For this review, take the finished solid that the model builds, in its own axes (mm). A direction names the side the tool comes from. Give positions to 0.01 mm unless a question says otherwise; leave off trailing zeros. Loops run counter-clockwise (first coordinate to the right, second up) from the corner with the lowest first, then second, coordinate; pieces in that order, holes last. Notation, with made-up numbers: (-1, 15) - (54, 15) arc R22 cw to (54, 27) - close; hole circle Ø11 at (-38, 72). An arc over 180 degrees is marked (long way). Answer in a Markdown table with one row per item.
Autodesk Inventor part; units mm, degrees
ref_plane "YZ Plane" through (0, 0, 0) normal (1, 0, 0) x (0, 1, 0)
ref_plane "XZ Plane" through (0, 0, 0) normal (0, 1, 0) x (-1, 0, 0)
ref_plane "XY Plane" through (0, 0, 0) normal (0, 0, 1) x (1, 0, 0)
sketch "Sketch1" plane through (0, 0, 0) normal (0, 0, 1) x (1, 0, 0)
  line L0 (91, -34) -> (91, 34)
  line L1 (91, 34) -> (41, 34)
  line L2 (41, 34) -> (41, 89)
  line L3 (41, 89) -> (-91, 89)
  line L4 (-91, 89) -> (-91, -89)
  line L5 (-91, -89) -> (41, -89)
  line L6 (41, -89) -> (41, -34)
  line L7 (41, -34) -> (91, -34)
  line L8 (70, 27) -> (62, 27)
  line L9 (91, 34) -> (-87, 34)
  line L10 (-87, 34) -> (-87, 27)
  line L11 (-87, 27) -> (91, 27)
  line L12 (91, 27) -> (91, 34)
  circle A0 centre (-83, 21.5) radius 1.2295
  circle A1 centre (-83, -64.5) radius 1.2295
  circle A2 centre (-83, -21.5) radius 1.2295
  circle A3 centre (-83, 64.5) radius 1.2295
  line L13 (-85, -72) -> (-76, -72)
  line L14 (-76, -72) -> (-76, -57)
  line L15 (-76, -57) -> (-85, -57)
  arc A4 (-87, -55) -> (-85, -57) centre (-85, -55) ccw
  line L16 (-87, -55) -> (-87, -31)
  arc A5 (-85, -29) -> (-87, -31) centre (-85, -31) ccw
  line L17 (-85, -29) -> (-76, -29)
  line L18 (-76, -29) -> (-76, -14)
  line L19 (-76, -14) -> (-85, -14)
  arc A6 (-87, -12) -> (-85, -14) centre (-85, -12) ccw
  line L20 (-87, -12) -> (-87, 12)
  arc A7 (-85, 14) -> (-87, 12) centre (-85, 12) ccw
  line L21 (-85, 14) -> (-76, 14)
  line L22 (-76, 14) -> (-76, 29)
  line L23 (-76, 29) -> (-85, 29)
  arc A8 (-87, 31) -> (-85, 29) centre (-85, 31) ccw
  line L24 (-87, 31) -> (-87, 55)
  arc A9 (-85, 57) -> (-87, 55) centre (-85, 55) ccw
  line L25 (-85, 57) -> (-76, 57)
  line L26 (-76, 57) -> (-76, 72)
  line L27 (-76, 72) -> (-85, 72)
  arc A10 (-87, 74) -> (-85, 72) centre (-85, 74) ccw
  line L28 (-87, 74) -> (-87, 89)
  line L29 (-91, 89) -> (-87, 89)
  line L30 (-91, -89) -> (-91, 89)
  line L31 (-91, -89) -> (-87, -89)
  line L32 (-87, -89) -> (-87, -74)
  arc A11 (-85, -72) -> (-87, -74) centre (-85, -74) ccw
  line L33 (-91, 89.5) -> (-86.5, 89.5)
  line L34 (-86.5, 89.5) -> (-86.5, 74)
  arc A12 (-86.5, 74) -> (-85, 72.5) centre (-85, 74) ccw
  line L35 (-85, 72.5) -> (-75.5, 72.5)
  line L36 (-75.5, 72.5) -> (-75.5, 56.5)
  line L37 (-75.5, 56.5) -> (-85, 56.5)
  arc A13 (-85, 56.5) -> (-86.5, 55) centre (-85, 55) ccw
  line L38 (-86.5, 55) -> (-86.5, 31)
  arc A14 (-86.5, 31) -> (-85, 29.5) centre (-85, 31) ccw
  line L39 (-85, 29.5) -> (-75.5, 29.5)
  line L40 (-75.5, 29.5) -> (-75.5, 13.5)
  line L41 (-75.5, 13.5) -> (-85, 13.5)
  arc A15 (-85, 13.5) -> (-86.5, 12) centre (-85, 12) ccw
  line L42 (-86.5, 12) -> (-86.5, -12)
  arc A16 (-86.5, -12) -> (-85, -13.5) centre (-85, -12) ccw
  line L43 (-85, -13.5) -> (-75.5, -13.5)
  line L44 (-75.5, -13.5) -> (-75.5, -29.5)
  line L45 (-75.5, -29.5) -> (-85, -29.5)
  arc A17 (-85, -29.5) -> (-86.5, -31) centre (-85, -31) ccw
  line L46 (-86.5, -31) -> (-86.5, -55)
  arc A18 (-86.5, -55) -> (-85, -56.5) centre (-85, -55) ccw
  line L47 (-85, -56.5) -> (-75.5, -56.5)
  line L48 (-75.5, -56.5) -> (-75.5, -72.5)
  line L49 (-75.5, -72.5) -> (-85, -72.5)
  arc A19 (-85, -72.5) -> (-86.5, -74) centre (-85, -74) ccw
  line L50 (-86.5, -74) -> (-86.5, -89.5)
  line L51 (-86.5, -89.5) -> (-91, -89.5)
  line L52 (-86.5, 31) -> (-75.5, 31)
  line L53 (-75.5, 31) -> (-75.5, 29.5)
  line L54 (-75.5, 31) -> (-75.5, 34)
  point P0 (0, 0)
  point P1 (-75.5, 27)
  point P2 (-86.5, 34)
  dimension "d6" = 0.5
extrude "Extrusion1" add sketch "Sketch1" along normal blind 30 contours L11 L8 L40 L53 L54 L9 L1 L0
sketch "Sketch3" plane through (-86.5, 34, 0) normal (0, 1, 0) x (1, 0, 0)
  line L0 (-0.5, -4.5) -> (-0.5, 0)
  line L1 (-0.5, 0) -> (-4.5, 0)
  line L2 (-4.5, 0) -> (-4.5, 3.5)
  line L3 (-4.5, 3.5) -> (-18.5, 3.5)
  line L4 (-18.5, 3.5) -> (-4.5, -5.5)
  line L5 (-4.5, -5.5) -> (-4.5, -4.5)
  line L6 (-4.5, -4.5) -> (-0.5, -4.5)
  line L7 (-0.5, -4.5) -> (50.0525, -33.6865)
  line L8 (177.5, 0) -> (11, 0)
  line L9 (177.5, -30) -> (11, -30)
  line L10 (177.5, 0) -> (177.5, -30)
  line L11 (11, 0) -> (11, -30)
  point P0 (86.5, 0)
  point P1 (43.6673, -30)
  point P2 (11, -11.1395)
  dimension "d7" = 30
extrude "Extrusion4" cut sketch "Sketch3" against normal blind 30 contours L7 L9 L11
sketch "Sketch5" plane through (-75.5, 27, 0) normal (0, -1, 0) x (1, 0, 0)
  line L0 (56.5, 7.0341) -> (57.5, 7.0341)
  line L1 (34.5, 7.0341) -> (56.5, 7.0341)
  line L2 (33.5, 7.0341) -> (33.5, 6.6226)
  line L3 (33.5, 6.6226) -> (9.5, 6.6226)
  line L4 (9.5, 6.6226) -> (9.5, 7.0341)
  line L5 (9.5, 7.0341) -> (33.5, 7.0341)
  line L6 (64.5, 7.0341) -> (64.5, 6.6226)
  line L7 (64.5, 6.6226) -> (57.5, 6.6226)
  line L8 (57.5, 6.6226) -> (57.5, 7.0341)
  line L9 (57.5, 7.0341) -> (64.5, 7.0341)
  line L10 (9.5, 2) -> (9.5, 2.6226)
  line L11 (9.5, 2.6226) -> (64.5, 2.6226)
  line L12 (64.5, 2.6226) -> (64.5, 2)
  line L13 (64.5, 2) -> (9.5, 2)
  line L14 (9.5, 7.0341) -> (64.5, 7.0341)
  line L15 (64.5, 7.0341) -> (64.5, 2)
  line L16 (64.5, 2) -> (9.5, 2)
  line L17 (9.5, 2) -> (9.5, 7.0341)
  line L18 (9.2, 7.3341) -> (64.8, 7.3341)
  line L19 (64.8, 7.3341) -> (64.8, 1.9)
  line L20 (64.8, 1.9) -> (9.2, 1.9)
  line L21 (9.2, 1.9) -> (9.2, 7.3341)
  point P0 (75.5, 0)
  dimension "d19" = 0.3
  dimension "d20" = 0.3
  dimension "d21" = 0.1
  dimension "d22" = 0.3
extrude "Extrusion6" cut sketch "Sketch5" against normal blind 0.7 contours L0 L8 L7 L15 L11 L17 L3 L2 L14 L1 | L9 L6 L7 L8 | L2 L3 L4 L5 | L12 L13 L10 L11 | L18 L19 L20 L21
sketch "Sketch6" plane through (-75.5, 27, 0) normal (0, -1, 0) x (1, 0, 0)
  line L0 (33.5, 7.0341) -> (34.5, 7.0341)
  line L1 (34.5, 7.0341) -> (56.5, 7.0341)
  line L2 (56.5, 7.0341) -> (57.5, 7.0341)
  line L3 (64.8, 1.9) -> (9.2, 1.9)
  line L4 (64.8, 7.3341) -> (64.8, 1.9)
  line L5 (9.2, 7.3341) -> (64.8, 7.3341)
  line L6 (9.2, 1.9) -> (9.2, 7.3341)
  line L7 (33.5, 7.3341) -> (57.5, 7.3341)
  line L8 (57.5, 7.3341) -> (57.5, 1.9)
  line L9 (57.5, 1.9) -> (33.5, 1.9)
  line L10 (33.5, 1.9) -> (33.5, 7.3341)
  point P0 (75.5, 0)
extrude "Extrusion7" cut sketch "Sketch6" against normal up to next contours L10 L5 L8 L2 L1 L0 | L0 L1 L2 L8 L3 L10
sketch "Sketch7" plane through (0, 0, 30) normal (0, 0, 1) x (1, 0, 0)
  line L0 (10.25, -34) -> (10.25, 34)
  line L1 (10.25, 34) -> (-5.75, 34)
  line L2 (-5.75, -34) -> (-5.75, 34)
  line L3 (10.25, -34) -> (-5.75, -34)
  line L4 (-42.8327, 27) -> (91, 27)
  line L5 (10.25, 34) -> (-5.75, 34)
  line L6 (-5.75, 34) -> (-5.75, 27)
  line L7 (-5.75, 27) -> (10.25, 27)
  line L8 (10.25, 27) -> (10.25, 34)
  line L9 (10.65, 34) -> (-6.15, 34)
  line L10 (-6.15, 34) -> (-6.15, 27)
  line L11 (-6.15, 27) -> (10.65, 27)
  line L12 (10.65, 27) -> (10.65, 34)
  point P0 (0, 0)
  dimension "d27" = 0.4
  dimension "d28" = 0.4
extrude "Extrusion8" cut sketch "Sketch7" against normal blind 15.5 contours L4 L2 L1 L0 | L0 L9 L12 L4 | L4 L10 L9 L2
properties part number "right_hold"
1. We need section B-B, the plane y = 32.75. Give the boundary of the cut face in (x, z).
Values:
| item | result |
|---|---|
| outline | (-75.5, 0) - (91, 0) - (91, 30) - (10.65, 30) - (10.65, 14.5) - (-6.15, 14.5) - (-6.15, 30) - (-42.83, 30) - (-75.5, 11.14) - close; hole (-42, 1.9) - (-18, 1.9) - (-18, 7.33) - (-42, 7.33) - close |
2. For faces 5 (the face through (-18, 31, 5)), 6 (the face through (-54, 27.7, 5)), 7 (the face through (50, 31, 30)), 8 (the face through (10.65, 30, 22)), list the 3-axis set-ups (+Z, -Z, +X, -X, +Y, -Y) from which the entire face can be reached by the end or side of a thin tool; tool diameter is ignored.
Values:
| item | result |
|---|---|
| face 5 | +Y, -Y |
| face 6 | -Y |
| face 7 | +Z, +X, -X, +Y, -Y |
| face 8 | +Z, +Y, -Y |
3. Clearance check with a flat-ended pin moving along its axis: pin 1 (1.6 mm diameter, centred on x = -13.5, z = 5.5, fed in from -Y). State where the tip first meets the part, or that it passes through.
Values:
| item | result |
|---|---|
| pin 1 | stops at y = 27.7 |
4. We need section C-C, the plane z = 17. Give the boundary of the cut face in (x, y).
Values:
| item | result |
|---|---|
| outline | (-65.35, 27) - (-6.15, 27) - (-6.15, 34) - (-65.35, 34) - close; (10.65, 27) - (91, 27) - (91, 34) - (10.65, 34) - close |
5. Mouldability with a two-part tool opening along Z and no side actions: class faces 1 (the face through (-14, 27.7, 5)), 2 (the face through (-6.15, 31, 22)), 3 (the face through (-59.395, 30.549, 20.438)), 4 (the face through (-33, 30, 7.334)) as released by +Z, released by -Z, zero draft, split by the parting line, or undercut.
Values:
| item | result |
|---|---|
| face 1 | undercut |
| face 2 | zero draft |
| face 3 | released by +Z |
| face 4 | undercut |
6. We need section A-A, the plane x = -31.5. Give the boundary of the cut face in (y, z).
Values:
| item | result |
|---|---|
| outline | (27, 0) - (34, 0) - (34, 1.9) - (27, 1.9) - close; (27, 7.33) - (34, 7.33) - (34, 30) - (27, 30) - close |
7. Wall thickness on line 1 (X direction, y = 30.25, z = 5.5); line 2 (Z direction, x = -37, y = 30.5); line 3 (Z direction, x = 5, y = 32.5): over which ranges is each line inside the solid? List them lowest first. Write a range as [from, to].
Values:
| item | result |
|---|---|
| line 1 | x = [-75.5, -42], [-18, 91] |
| line 2 | z = [0, 1.9], [7.33, 30] |
| line 3 | z = [0, 14.5] |
